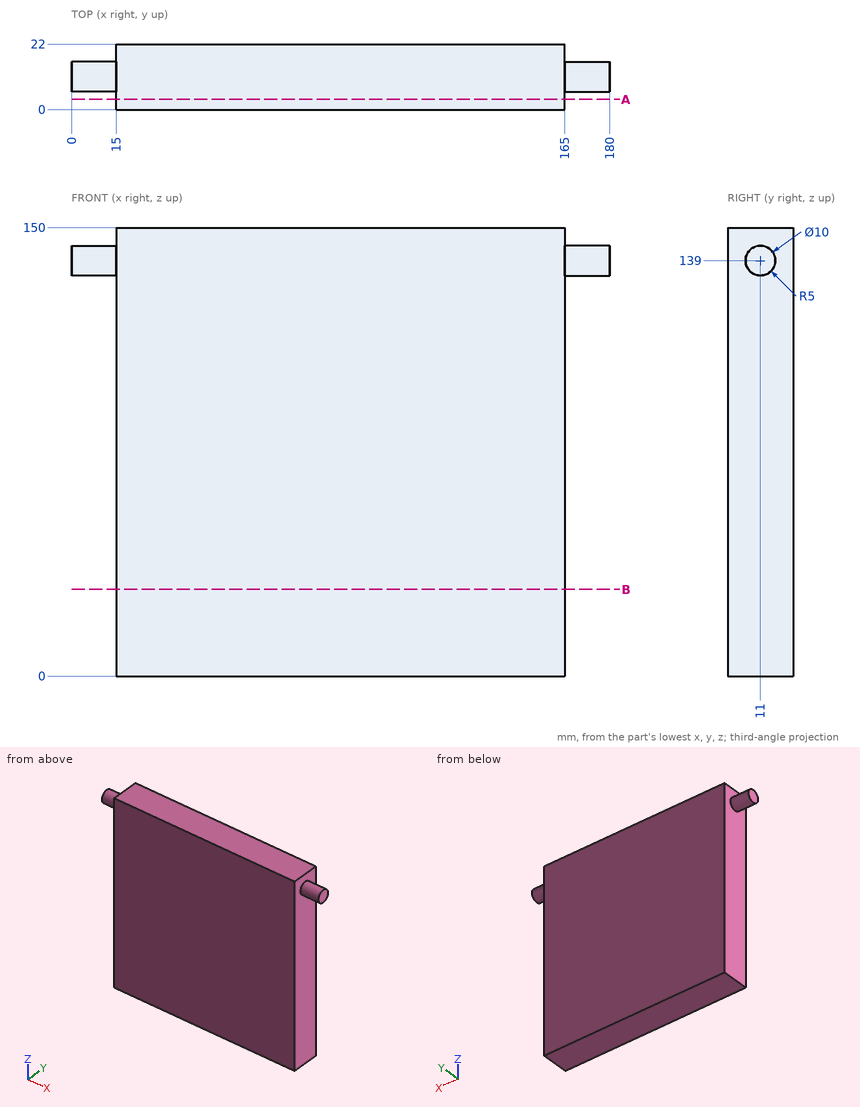
Geometry: see drawing. Coordinates: mm, zero at the bounding-box minimum. Coordinates: 2 decimals unless noted, no trailing zeros. Write each loop counter-clockwise with the first axis right and the second up, starting at its lowest first coordinate (ties: lowest second). Pieces come first, ordered by that corner, then holes.
1) Material intervals for line 1 along X through (y, z) = (7.5, 96); line 2 along Z through (x, y) = (170, 12.75), sorted ascending.
2) Section A-A on y = 3.5. Output: boundary loops of the cut face in (x, z).
3) Section B-B on z = 29. Output: boundary loops of the cut face in (x, y), and give its area (3 significant figures).
4) Pin query (flat end, axial travel): pin 1 Ø5 at (x, z) = (143, 25.5) entering from -Y; pin 2 Ø11 at (y, z) = (5.5, 46.5) entering from -X; pin 3 Ø8 at (y, z) = (16.5, 93) entering from +X. Return the tip coordinate at first contact, or that it passes through.
Check result:
1. line 1: x = 15 to 165
1. line 2: z = 134.32 to 143.68
2. outline: (15, 0) - (165, 0) - (165, 150) - (15, 150) - close
3. outline: (15, 0) - (165, 0) - (165, 22) - (15, 22) - close
3. area: 3,300 mm2
4. pin 1: stops at y = 0
4. pin 2: stops at x = 15
4. pin 3: stops at x = 165
